Input: dimensioned drawing with shaded views. Units: mm. Origin: part minimum x, y, z. Coordinates: 2 decimals unless noted, no trailing zeros. Loops run counter-clockwise (first coordinate to the right, second up) from the corner with the lowest first, then second, coordinate; pieces in that order, holes last. Notation, with made-up numbers: (-20.75, 48.5) - (20.25, 48.5) arc R20 cw to (20.25, 59.5) - close; hole circle Ø5 at (31, 79). An arc over 180 degrees is marked (long way). Use one line per item in the form item = value. Start each with the question number.
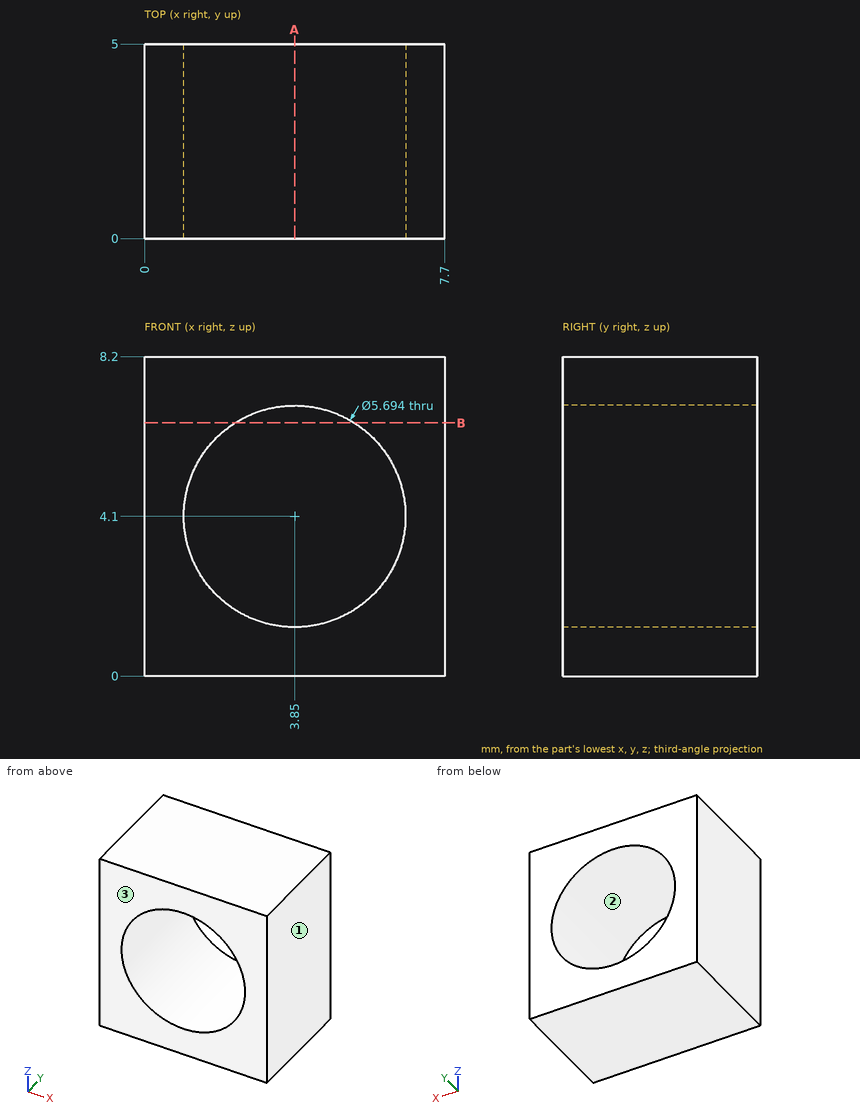
(1) Contact query for a flat-ended pin moving along its axis: pin 1 (4.5 mm diameter, centred on x = 3.85, z = 4.1, fed in from -Y). Output: stop coordinate, or through.
(2) Mould query, pull axis X, two halves, no side actions, for the marked faces 1, 2 and 3. Classes: +X half, -X half, draft (parallel to the pull), parting line (faces both ways), or undercut.
(3) Cut plane B-B, the plane z = 6.5. Output: boundary loops of the cut face in (x, y).
(4) Material intervals for line 1 (Z direction, x = 3.85, y = 1.9); line 2 (Z direction, x = 2.5, y = 2.45); line 3 (X direction, y = 1.15, z = 5.5), sorted ascending.
(5) Cut plane A-A, the plane x = 3.85. Output: boundary loops of the cut face in (y, z).
Recorded:
q1.pin_1 = through
q2.face_1 = +X half
q2.face_2 = undercut
q2.face_3 = draft
q3.outline = (0, 0) - (2.32, 0) - (2.32, 5) - (0, 5) - close; (5.38, 0) - (7.7, 0) - (7.7, 5) - (5.38, 5) - close
q4.line_1 = 0 to 1.25, 6.95 to 8.2
q4.line_2 = 0 to 1.59, 6.61 to 8.2
q4.line_3 = 0 to 1.37, 6.33 to 7.7
q5.outline = (0, 0) - (5, 0) - (5, 1.25) - (0, 1.25) - close; (0, 6.95) - (5, 6.95) - (5, 8.2) - (0, 8.2) - close
